Here's the drawing with two shaded views (mm, measured from the low corner). I have some questions. A direction names the side the tool comes from. Give positions to 0.01 mm unless a question says otherwise; leave off trailing zeros. Write each loop counter-clockwise with the first axis right and the second up, starting at its lowest first coordinate (ties: lowest second). Pieces come first, ordered by that corner, then holes. Notation, with made-up numbers: (-28.5, 70) - (8.5, 70) arc R8 cw to (8.5, 75) - close; hole circle Ø4 at (78.5, 8). An arc over 180 degrees is marked (long way). Answer as a JSON object with one key per item and string values. Group by question number.
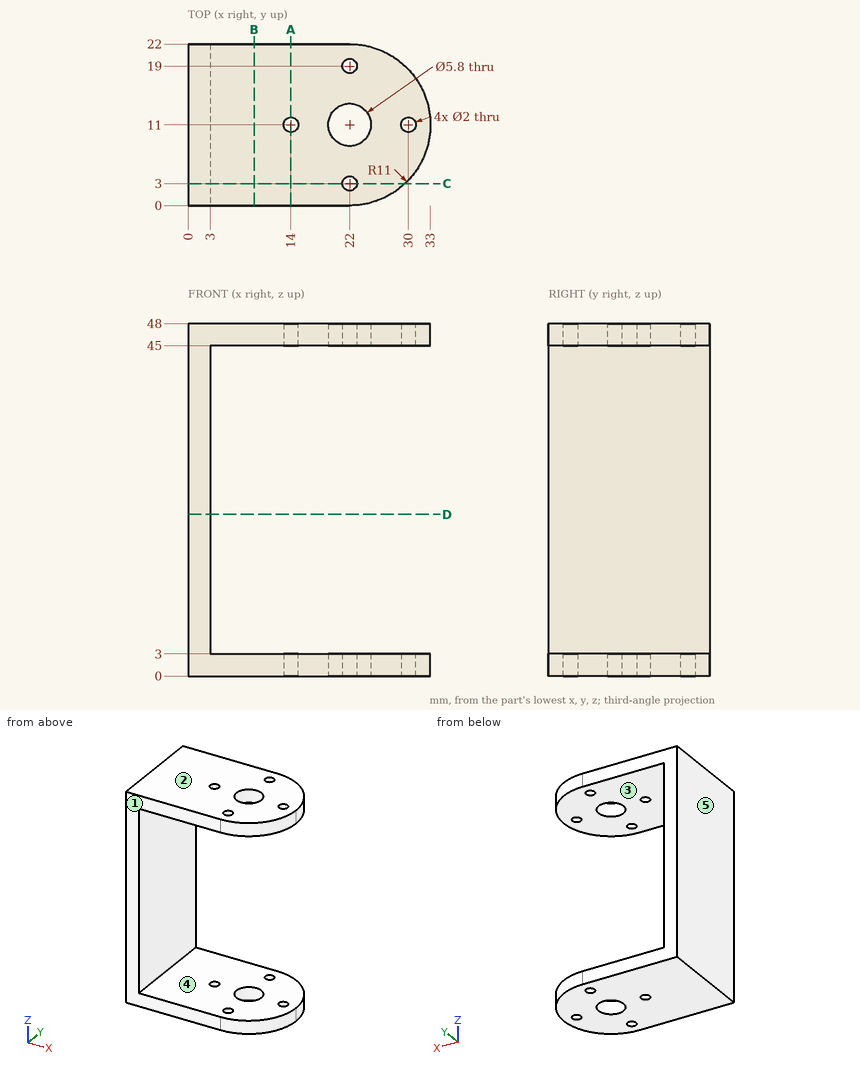
(1) Will these pins go through, and if not, where does the flat tip stop? P1, Ø1.2, axis at x = 30, y = 11, coming from the +Z side; P2, Ø4, axis at y = 15, z = 9.5, coming from the +X side.
(2) I want a section at B-B, the plane x = 9. Please give me the cut outline in (y, z).
(3) I want a section at D-D, the plane z = 22. Please give me the cut outline in (x, y), and give its area (3 significant figures).
(4) I want a section at C-C, the plane y = 3. Please give me the cut outline in (x, z), and give its area (3 significant figures).
(5) For the marked faces 4 and 5, which set-ups out of +Z, -Z, +X, -X, +Y, -Y let a thin tool reach every point of the face, with its end or its side?
(6) I want a section at A-A, the plane x = 14. Please give me the cut outline in (y, z), and give its area (3 significant figures).
(7) If we mould it in two halves opening along Z, with no side actions, what happens to the marked faces 1, 2 and 3? For each: +Z half, -Z half, draft (parallel to the pull), parting line (faces both ways), or undercut.
(8) I need wall thicknesses on L1, parallel to X at y = 11, z = 46.7; L2, parallel to Y at x = 22, z = 46.2; L3, parallel to Z at x = 30, y = 12.5. Which ranges of each line are inside material? Lowest first, please.
Entries:
{
 "1": {"P1": "through", "P2": "x = 3"},
 "2": {"outline": "(0, 0) - (22, 0) - (22, 3) - (0, 3) - close; (0, 45) - (22, 45) - (22, 48) - (0, 48) - close"},
 "3": {"outline": "(0, 0) - (3, 0) - (3, 22) - (0, 22) - close", "area": "66.0 mm^2"},
 "4": {"outline": "(0, 0) - (21, 0) - (21, 3) - (3, 3) - (3, 45) - (21, 45) - (21, 48) - (0, 48) - close; (23, 0) - (29.55, 0) - (29.55, 3) - (23, 3) - close; (23, 45) - (29.55, 45) - (29.55, 48) - (23, 48) - close", "area": "291 mm^2"},
 "5": {"face 4": "+X, +Y, -Y", "face 5": "+Z, -Z, -X, +Y, -Y"},
 "6": {"outline": "(0, 0) - (10, 0) - (10, 3) - (0, 3) - close; (0, 45) - (10, 45) - (10, 48) - (0, 48) - close; (12, 0) - (22, 0) - (22, 3) - (12, 3) - close; (12, 45) - (22, 45) - (22, 48) - (12, 48) - close", "area": "120 mm^2"},
 "7": {"face 1": "draft", "face 2": "+Z half", "face 3": "undercut"},
 "8": {"L1": "0 to 13, 15 to 19.1, 24.9 to 29, 31 to 33", "L2": "0 to 2, 4 to 8.1, 13.9 to 18, 20 to 22", "L3": "0 to 3, 45 to 48"}
}
